from build123d import *

# Parameters (mm, degrees)
SKETCH1_R           = 37.25
BOSS_EXTRUDE1_DEPTH = 8
SKETCH2_R           = 8
SKETCH2_R_2         = 6
BOSS_EXTRUDE2_DEPTH = 60
CHAMFER1_SIZE       = 3
CUT_EXTRUDE1_START  = -10
SKETCH3_R           = 6
CUT_EXTRUDE1_DEPTH  = 10
SKETCH4_R           = 2.25
CUT_EXTRUDE2_DEPTH  = 10


with BuildPart() as part:
    # Sketch1 → Boss-Extrude1 (new body)
    with BuildSketch(Plane(origin=(0, 0, 0), x_dir=(1, 0, 0), z_dir=(0, 1, 0))):
        with Locations(Location((0, 0, 0), (0, 0, 270))):
            Circle(SKETCH1_R)
    extrude(amount=BOSS_EXTRUDE1_DEPTH)

    # Sketch2 → Boss-Extrude2 (add)
    with BuildSketch(Plane(origin=(0, 8, 0), x_dir=(1, 0, 0), z_dir=(0, 1, 0))):
        with Locations(Location((0, 0, 0), (0, 0, 270))):
            Circle(SKETCH2_R)
        with Locations(Location((0, 0, 0), (0, 0, 270))):
            Circle(SKETCH2_R_2, mode=Mode.SUBTRACT)
    extrude(amount=BOSS_EXTRUDE2_DEPTH)

    # Chamfer1
    chamfer1_edges = [part.edges().sort_by_distance(p)[0] for p in [
        (0, 8, -37.25),
    ]]
    chamfer(chamfer1_edges, length=CHAMFER1_SIZE)

    # Sketch3 → Cut-Extrude1 (cut)
    with BuildSketch(Plane(origin=(0, 8, 0), x_dir=(1, 0, 0), z_dir=(0, 1, 0)).offset(CUT_EXTRUDE1_START)):
        with Locations(Location((0, 0, 0), (0, 0, 270))):
            Circle(SKETCH3_R)
    extrude(amount=CUT_EXTRUDE1_DEPTH, mode=Mode.SUBTRACT)

    # Sketch4 → Cut-Extrude2 (cut)
    with BuildSketch(Plane(origin=(0, 0, 0), x_dir=(-1, 0, 0), z_dir=(0, -1, 0))):
        with Locations(Location((20.506096654, 20.506096654, 0), (0, 0, 90))):
            Circle(SKETCH4_R)
        with Locations(Location((20.506096654, -20.506096654, 0), (0, 0, 90))):
            Circle(SKETCH4_R)
        with Locations(Location((-20.506096654, -20.506096654, 0), (0, 0, 90))):
            Circle(SKETCH4_R)
        with Locations(Location((-20.506096654, 20.506096654, 0), (0, 0, 90))):
            Circle(SKETCH4_R)
        with BuildLine():
            ThreePointArc((29.777070039, -14.224137931), (33, 0), (29.777070039, 14.224137931))
            ThreePointArc((29.777070039, 14.224137931), (24.443590285, 16.109341823), (22.558386393, 10.775862069))
            ThreePointArc((22.558386393, 10.775862069), (25, 0), (22.558386393, -10.775862069))
            ThreePointArc((22.558386393, -10.775862069), (24.443590285, -16.109341823), (29.777070039, -14.224137931))
        make_face()
        with BuildLine():
            ThreePointArc((-14.224137931, -29.777070039), (0, -33), (14.224137931, -29.777070039))
            ThreePointArc((14.224137931, -29.777070039), (16.109341823, -24.443590285), (10.775862069, -22.558386393))
            ThreePointArc((10.775862069, -22.558386393), (0, -25), (-10.775862069, -22.558386393))
            ThreePointArc((-10.775862069, -22.558386393), (-16.109341823, -24.443590285), (-14.224137931, -29.777070039))
        make_face()
        with BuildLine():
            ThreePointArc((14.224137931, 29.777070039), (0, 33), (-14.224137931, 29.777070039))
            ThreePointArc((-14.224137931, 29.777070039), (-16.109341823, 24.443590285), (-10.775862069, 22.558386393))
            ThreePointArc((-10.775862069, 22.558386393), (0, 25), (10.775862069, 22.558386393))
            ThreePointArc((10.775862069, 22.558386393), (16.109341823, 24.443590285), (14.224137931, 29.777070039))
        make_face()
    extrude(amount=-CUT_EXTRUDE2_DEPTH, mode=Mode.SUBTRACT)


solid = part.part
Verification items for the finished model (mm, model axes). A direction names the side the tool comes from. Coordinates: 2 decimals unless noted, no trailing zeros. Order: outer loops, then holes, each group sorted by start corner. A loop starts at its lowest first (then second) coordinate and runs counter-clockwise, first axis right, second up.
1. Sectioned sample at A-A, the plane x = 0. Record the cut outline in (y, z).
Results found:
outline: (0, -37.25) - (5, -37.25) - (8, -34.25) - (8, -33) - (0, -33) - close; (0, -25) - (8, -25) - (8, -8) - (68, -8) - (68, -6) - (0, -6) - close; (0, 6) - (68, 6) - (68, 8) - (8, 8) - (8, 25) - (0, 25) - close; (0, 33) - (8, 33) - (8, 34.25) - (5, 37.25) - (0, 37.25) - close
2. Set-up check for faces 1 (the face through (6, 68, -2)), 2 (the face through (-7.81, 37.58, -1.73)), 3 (the face through (0, 4, -25)): record each of +Z, -Z, +X, -X, +Y, -Y from which the full face is reachable in a straight line by a thin tool's end or side.
Results found:
face 1: +Z, -Z, +X, -X, +Y
face 2: +Y
face 3: +Y, -Y
3. Sectioned sample at B-B, the plane y = 19. Record the cut outline in (x, z).
Results found:
outline: circle Ø16 at (0, 0); hole circle Ø12 at (0, 0)
4. Sectioned sample at C-C, the plane z = 2.5. Give the number of separate pieces and of enclosed holes in the cut face, and give its area (3 significant figures).
Results found:
separate pieces: 3
enclosed holes: 0
area: 692 mm2
5. Go/stop test with flat-tipped pins: pin 1 Ø10 at (y, z) = (22, 15) entering from -X; pin 2 Ø6 at (x, z) = (3, 13) entering from +Y; pin 3 Ø10 at (y, z) = (39, 5) entering from +X; pin 4 Ø6 at (y, z) = (26, 10) entering from -X. Record where each tip stops, or that it passes through.
Results found:
pin 1: passes through
pin 2: stops at y = 8
pin 3: stops at x = 8
pin 4: stops at x = -3.87
6. Scan lines: line 1 (Y direction, x = -21.5, z = -18); line 2 (X direction, y = 16, z = -1); line 3 (Z direction, x = 4.5, y = 12.5). Record each from-to range of solid material in increasing order.
Results found:
line 1: y = 0 to 8
line 2: x = -7.94 to -5.92, 5.92 to 7.94
line 3: z = -6.61 to -3.97, 3.97 to 6.61
7. Release check for a two-part mould opening along Z. For faces 4 (the face through (10.33, 7.85, 32.81)), 5 (the face through (8, 8, 7)), 6 (the face through (-22.502, 3.944, 19.468)) record: +Z half, -Z half, draft (parallel to the pull), parting line (faces both ways), or undercut.
Results found:
face 4: parting line
face 5: draft
face 6: undercut
